Work out the finished part from the listing and answer in its coordinate system (mm). A direction names the side the tool comes from. Coordinates: 2 decimals unless noted, no trailing zeros. Loops run counter-clockwise (first coordinate to the right, second up) from the corner with the lowest first, then second, coordinate; pieces in that order, holes last. Notation, with made-up numbers: (79, -9.5) -> (117, -9.5) arc R28 ccw to (117, 10.5) -> close; hole circle Ø7 at (6.5, 21). An arc over 180 degrees is marked (long way). Answer as CSV lines item,"result".
```python
from build123d import *

# Parameters (mm, degrees)
PAD028_DEPTH  = 1
SKETCH038_R   = 2.1
HOLE001_DEPTH = 25
PAD027_DEPTH  = 17


with BuildPart() as part:
    # Sketch037 (on Face1 of CopyPad003) → Pad028 (new body)
    with BuildSketch(Plane.XY.offset(19)):
        with BuildLine():
            ThreePointArc((-13.555442, -3.5), (0, -14), (13.555442, -3.5))
            Line((13.555442, -3.5), (17.5, -3.5))
            ThreePointArc((17.5, -3.5), (21, 0), (17.5, 3.5))
            Line((13.555442, 3.5), (17.5, 3.5))
            ThreePointArc((13.555442, 3.5), (0, 14), (-13.555442, 3.5))
            Line((-13.555442, 3.5), (-17.5, 3.5))
            ThreePointArc((-17.5, 3.5), (-21, 0), (-17.5, -3.5))
            Line((-13.555442, -3.5), (-17.5, -3.5))
        make_face()
    extrude(amount=-PAD028_DEPTH)

    # Sketch038 (on Face9 of Pad028) → Hole001 (cut)
    with BuildSketch(Plane.XY.offset(19)):
        with Locations((-17.5, 0)):
            Circle(SKETCH038_R)
        with Locations((17.5, 0)):
            Circle(SKETCH038_R)
    extrude(amount=-HOLE001_DEPTH, mode=Mode.SUBTRACT)

    # Sketch006 (on Face4 of Hole001) → Pad027 (join)
    with BuildSketch(Plane.XY.offset(19)):
        with BuildLine():
            Line((-7.3, -11), (7.3, -11))
            Line((7.3, -11), (7.3, -16))
            ThreePointArc((6.3, -17), (7.007107, -16.707107), (7.3, -16))
            Line((6.3, -17), (-6.3, -17))
            ThreePointArc((-7.3, -16), (-7.007107, -16.707107), (-6.3, -17))
            Line((-7.3, -16), (-7.3, -11))
        make_face()
    extrude(amount=-PAD027_DEPTH)


solid = part.part
```
(1) A cutting plane is placed at B-B, the plane z = 6.5. Write down the section's boundary in (x, y).
Computed values:
outline,"(-7.3, -16) arc R1 ccw to (-6.3, -17) -> (6.3, -17) arc R1 ccw to (7.3, -16) -> (7.3, -11) -> (-7.3, -11) -> close"
(2) Which of the six approach directions +Z, -Z, +X, -X, +Y, -Y give full straight-line access (tool end or side, diameter ignored) to faces 1 (the face through (0, -11, 10)), 2 (the face through (15.5, -3.5, 18.5)), 3 (the face through (-21, 0.1, 18.5)), 4 (the face through (-15.5, -3.5, 18.5)), 5 (the face through (15.5, 3.5, 18.5))?
Computed values:
face 1,"-Z, +X, -X, +Y"
face 2,"+Z, -Z, +X, -Y"
face 3,"+Z, -Z, -X"
face 4,"+Z, -Z, -X, -Y"
face 5,"+Z, -Z, +X, +Y"
(3) For a pull along Y with two mould halves and no side action, classify faces 6 (the face through (-15.497, 0.631, 18.507)), 7 (the face through (-15.5, 3.5, 18.5)), 8 (the face through (0, 1, 18)) as pulls with the +Y half, pulls with the -Y half, needs draft (parallel to the pull), parting line crosses it, or undercut.
Computed values:
face 6,"undercut"
face 7,"pulls with the +Y half"
face 8,"needs draft"
(4) A cutting plane is placed at D-D, the plane y = -15. Write down the section's boundary in (x, z), and give its area (3 significant figures).
Computed values:
outline,"(-7.3, 2) -> (7.3, 2) -> (7.3, 19) -> (-7.3, 19) -> close"
area,"248 mm2"
(5) A cutting plane is placed at A-A, the plane y = 0. Write down the section's boundary in (x, z), and give its area (3 significant figures).
Computed values:
outline,"(-21, 18) -> (-19.6, 18) -> (-19.6, 19) -> (-21, 19) -> close; (-15.4, 18) -> (15.4, 18) -> (15.4, 19) -> (-15.4, 19) -> close; (19.6, 18) -> (21, 18) -> (21, 19) -> (19.6, 19) -> close"
area,"33.6 mm2"
(6) A cutting plane is placed at C-C, the plane x = -14.5. Write down the section's boundary in (y, z), and give its area (3 significant figures).
Computed values:
outline,"(-3.5, 18) -> (3.5, 18) -> (3.5, 19) -> (-3.5, 19) -> close"
area,"7.00 mm2"
(7) Consider line 1 along Y through (x, z) = (17.5, 18.3); line 2 along Y through (x, z) = (-3, 7); line 3 along Z through (x, y) = (-3, -5). Determine where each line is inside the solid, lowest interval first.
Computed values:
line 1,"-3.5 to -2.1, 2.1 to 3.5"
line 2,"-17 to -11"
line 3,"18 to 19"
(8) Flat-ended cylindrical pins translate along their axes: pin 1 Ø3.5 at (x, y) = (17.5, 0) entering from -Z; pin 2 Ø5 at (x, z) = (-10, 17) entering from +Y; pin 3 Ø6 at (x, y) = (-1.5, 1) entering from -Z; pin 4 Ø4 at (y, z) = (-13, 8.5) entering from -X. Find the tip coordinate at first contact, or state that the pin passes through.
Computed values:
pin 1,"through"
pin 2,"y = 11.69"
pin 3,"z = 18"
pin 4,"x = -7.3"
